Verification items for the finished model (mm, model axes). Face numbers are marked on the shaded views. Coordinates: 2 decimals unless noted, no trailing zeros. Order: outer loops, then holes, each group sorted by start corner. A loop starts at its lowest first (then second) coordinate and runs counter-clockwise, first axis right, second up.
Q1. Depth check by flat-ended pin: P1, Ø2, axis at y = -125.5, z = -217, coming from the -X side; P2, Ø3, axis at y = -125.5, z = -234.5, coming from the +X side; P3, Ø1, axis at y = -93.5, z = 105, coming from the +X side. Enter the tip coordinate at first touch or a pass-through.
Q2. Draft check along Z on the marked faces 1, 2 and 3. Enter one of: pulls with the +Z half, pulls with the -Z half, needs draft (parallel to the pull), parting line crosses it, or undercut.
Q3. Thickness scan on line 1 (Z direction, x = 0, y = -125); line 2 (Z direction, x = 46, y = -63); line 3 (Y direction, x = -53, z = -152.5). Record the ranges inside material, lowest first.
Q4. Cross-section at A-A, the plane x = 0. Record the boundary of the cut face in (y, z), and give its area (3 significant figures).
from build123d import *

# Parameters (mm, degrees)
F0_DEPTH = 127.137767151
F8_R     = 30.5052612997
F9_W     = 130
F9_H     = 65
F1_DEPTH = 404.413504526
F2_R     = 13.6095495466
F3_T     = -2.5
F5_D     = 50


with BuildPart() as f0:
    # F7 (on Front) → F0 (new body)
    with BuildSketch(Plane.XZ):
        with BuildLine():
            add(Edge.make_bspline(
                [(125, 250), (96.1666926742, 166.6666666667), (38.5000792642, 0), (96.1666901906, -166.6666666667), (125, -250)],
                knots=[0, 0, 0, 0, 0.5, 1, 1, 1, 1], degree=3))
            Line((125, 250), (-125, 250))
            Line((-125, 250), (-125, -250))
            Line((-125, -250), (125, -250))
        make_face()
    extrude(amount=F0_DEPTH)

    # F8
    f8_edges = [f0.edges().sort_by_distance(p)[0] for p in [
        (67.333385, -127.137767, 0),
        (-125, -127.137767, 0),
    ]]
    fillet(f8_edges, radius=F8_R)

    # F9 (on face) → F1 (cut)
    with BuildSketch(Plane(origin=(0, 0, 0), x_dir=(-1, 0, 0), z_dir=(0, 1, 0))):
        with Locations((20, -217.5)):
            Rectangle(F9_W, F9_H)
    extrude(amount=-F1_DEPTH, mode=Mode.SUBTRACT)

    # F2
    f2_edges = [f0.edges().sort_by_distance(p)[0] for p in [
        (45, -63.568884, -185),
        (-85, -63.568884, -185),
    ]]
    fillet(f2_edges, radius=F2_R)

    # F3
    f3_openings = [f0.faces().sort_by_distance(p)[0] for p in [
        (-17.051006, 0, 18.486444),
        (-20, -63.568884, -185),
        (-81.013855, -63.568884, -188.986145),
        (41.013855, -63.568884, -188.986145),
        (84.304295, -62.364714, -250),
        (-104.461032, -61.249084, -250),
        (-85, -63.568884, -224.304775),
        (45, -63.568884, -224.304775),
    ]]
    offset(amount=F3_T, openings=f3_openings, kind=Kind.INTERSECTION)

    # F5 (through all)
    with Locations(Plane.XZ.offset(127.137767151)):
        with Locations((0, 180.3100854158), (0, -123.9344850183)):
            Hole(F5_D / 2)


solid = f0.part
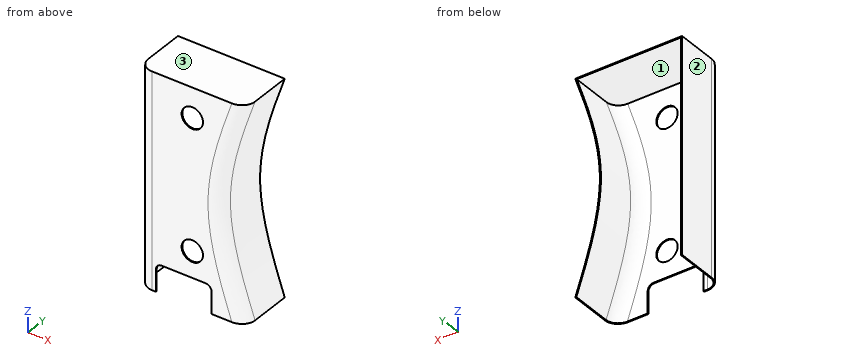
Check values:
1. P1: stops at x = -106.9
1. P2: stops at x = 101.67
1. P3: stops at x = 80.57
2. face 1: undercut
2. face 2: needs draft
2. face 3: pulls with the +Z half
3. line 1: z = -185 to -148.93, -98.93 to 155.31, 205.31 to 250
3. line 2: z = 247.5 to 250
3. line 3: y = -127.14 to -124.64
4. outline: (-127.14, -185) - (-124.64, -185) - (-124.64, -148.93) - (-127.14, -148.93) - close; (-127.14, -98.93) - (-124.64, -98.93) - (-124.64, 155.31) - (-127.14, 155.31) - close; (-127.14, 205.31) - (-124.64, 205.31) - (-124.64, 247.5) - (0, 247.5) - (0, 250) - (-127.14, 250) - close
4. area: 1,150 mm2
